Design review of the part built by this model. Coordinates are the model's own, in mm. A direction names the side the tool comes from. Give positions to 0.01 mm unless a question says otherwise; leave off trailing zeros. Order: outer loops, then holes, each group sorted by start corner. A loop starts at its lowest first (then second) coordinate and runs counter-clockwise, first axis right, second up. Notation, with made-up numbers: (56, -27) -> (77, -27) arc R10 ccw to (77, -17) -> close; hole circle Ø3 at (-6.75, -16). An arc over 180 degrees is marked (long way). Return JSON: item names as keys, results as strings.
```python
from build123d import *

# Parameters (mm, degrees)
BOSS_EXTRUDE1_DEPTH = 3
SKETCH2_W           = 130
SKETCH2_H           = 40
BOSS_EXTRUDE2_DEPTH = 12
CUT_EXTRUDE1_REACH  = 199.041
FILLET1_R           = 10
FILLET2_R           = 4


with BuildPart() as part:
    # Sketch1 → Boss-Extrude1 (new body)
    with BuildSketch(Plane.XY):
        with BuildLine():
            Line((190, 0), (190, -39))
            Line((190, -39), (0, -39))
            Line((0, -39), (0, 0))
            ThreePointArc((0, 0), (95, 50), (190, 0))
        make_face()
    extrude(amount=BOSS_EXTRUDE1_DEPTH)

    # Sketch2 → Boss-Extrude2 (add)
    with BuildSketch(Plane.XY.offset(3)):
        with Locations((95, -9)):
            Rectangle(SKETCH2_W, SKETCH2_H)
    extrude(amount=BOSS_EXTRUDE2_DEPTH)

    # Sketch3 → Cut-Extrude1 (cut, up to next)
    with BuildSketch(Plane(origin=(0, 11, 0), x_dir=(1, 0, 0), z_dir=(0, 1, 0)), mode=Mode.PRIVATE) as cut_extrude1_sk1:
        with BuildLine():
            Line((30, -15), (160, -15))
            ThreePointArc((160, -15), (95, -4.241357564), (30, -15))
        make_face()
    cut_extrude1_tool1 = extrude(cut_extrude1_sk1.sketch, amount=-CUT_EXTRUDE1_REACH, mode=Mode.PRIVATE) & part.part
    add(cut_extrude1_tool1.solids().sort_by_distance((95, 11, 10.686553))[0], mode=Mode.SUBTRACT)

    # Fillet1
    # the kernel refuses this fillet: 10 mm, written as the material it takes off along each edge
    with BuildSketch(Plane(origin=(160, 43.655354589, 15), x_dir=(0, 0, -1), z_dir=(0, -1, 0)), Plane(origin=(30, -61.655354589, 15), x_dir=(0, 0, -1), z_dir=(0, 1, 0))) as fillet1_piece_1:
        with BuildLine():
            CenterArc((13.461551545, -9.892616796), FILLET1_R, 98.40417735, 96.681797386)
            Line((3.806187845, -12.495298453), (3.613080571, -12.547352086))
            ThreePointArc((3.613080571, -12.547352086), (1.812932851, -6.275113154), (-0.189333785, -0.064441584))
            Line((-0.189333785, -0.064441584), (0, 0.2))
            ThreePointArc((0, 0.2), (6, 0.2), (11.970768969, 0.197852336))
            Line((11.970768969, 0.197852336), (12, 0))
        make_face()
    extrude(amount=105.310709179, mode=Mode.SUBTRACT)

    # Fillet2
    fillet2_edges = [part.edges().sort_by_distance(p)[0] for p in [
        (95, -29, 4.241357564),
        (95, 11, 4.241357564),
        (34.408965823, 11, 9.900838783),
        (155.591034177, 11, 9.900838783),
        (34.408965823, -29, 9.900838783),
        (155.591034177, -29, 9.900838783),
    ]]
    fillet(fillet2_edges, radius=FILLET2_R)


solid = part.part
```
Item 1: Add section C-C (y = 36.5). Give the boundary of the cut face in (x, z).
Result set:
{"outline": "(40.88, 0) -> (149.12, 0) -> (149.12, 3) -> (40.88, 3) -> close"}
Item 2: Add section B-B (x = 16). Give the boundary of the cut face in (y, z), plus the area to 3 significant figures.
Result set:
{"outline": "(-39, 0) -> (18.66, 0) -> (18.66, 3) -> (-39, 3) -> close", "area": "173 mm^2"}
Item 3: Wall thickness on L1, parallel to Z at x = 23.5, y = -19.5; L2, parallel to Z at x = 97, y = -7.5; L3, parallel to X at y = 3, z = 1.25: over which ranges is each line inside the solid? List them lowest first. Write a range as [from, to].
Result set:
{"L1": "z = [0, 3]", "L2": "z = [0, 4.25]", "L3": "x = [2.13, 187.87]"}
Item 4: Mouldability with a two-part tool opening along X and no side actions: class faces 1 (the face through (145, 11, 5)), 2 (the face through (93.44, 49.99, 1.48)), 3 (the face through (95.744, -8.761, 4.243)) as released by +X, released by -X, zero draft, split by the parting line, or undercut.
Result set:
{"face 1": "zero draft", "face 2": "split by the parting line", "face 3": "undercut"}
Item 5: Add section A-A (y = -19). Give the boundary of the cut face in (x, z).
Result set:
{"outline": "(0, 0) -> (190, 0) -> (190, 3) -> (160, 3) arc R10 ccw to (147.5, 11.19) arc R201.73 cw to (42.5, 11.19) arc R10 ccw to (30, 3) -> (0, 3) -> close"}
Item 6: For pin 1 (3.5 mm diameter, centred on x = 45.5, z = 6.5, fed in from -Y); pin 2 (2 mm diameter, centred on y = 12.5, z = 4.5, fed in from -X); pin 3 (10 mm diameter, centred on x = 23.5, y = 3, fed in from -Z); pin 4 (1.4 mm diameter, centred on x = 145.5, z = 6, fed in from +Y), all flat-tipped, find the tip position at first contact; note any pin that passes through.
Result set:
{"pin 1": "stops at y = -29", "pin 2": "passes through", "pin 3": "stops at z = 0", "pin 4": "stops at y = 11"}
Item 7: Machinability: for faces 4 (the face through (45, 11, 5)), 5 (the face through (45, -29, 5)), 6 (the face through (96, -4, 0)), which of the approach directions +Z, -Z, +X, -X, +Y, -Y give a long, thin tool a straight path to every point of the face, cutting with its end or side? Answer none if there is none.
Result set:
{"face 4": "+Z, +X, -X, +Y", "face 5": "+Z, +X, -X, -Y", "face 6": "-Z, +X, -X, +Y, -Y"}
